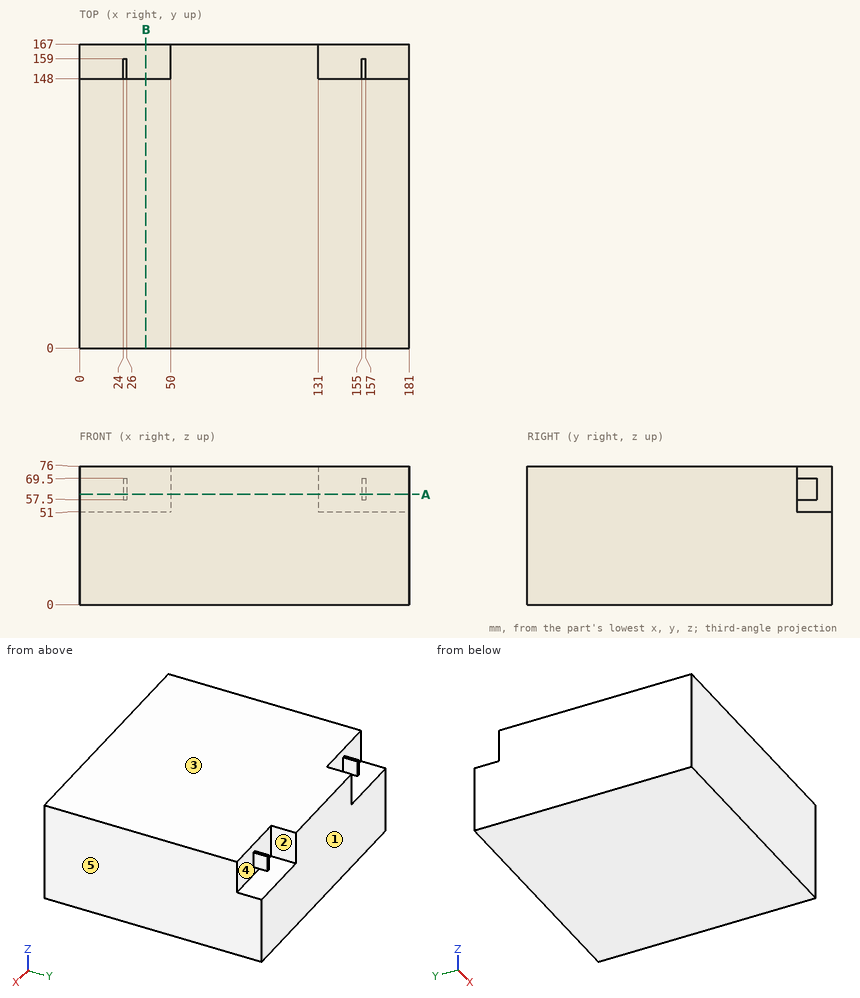
Geometry: see drawing. Coordinates: mm, zero at the bounding-box minimum. A direction names the side the tool comes from. Give positions to 0.01 mm unless a question says otherwise; leave off trailing zeros. Write each loop counter-clockwise with the first axis right and the second up, starting at its lowest first coordinate (ties: lowest second). Pieces come first, ordered by that corner, then holes. Notation, with made-up numbers: M 76,-8 L 117,-8 A17 ccw 117,-3 Z; hole C -32,-15.75 d2. An arc over 180 degrees is marked long. Return JSON: item names as keys, results as strings. Group by question number.
1) Set-up query: the marked faces 1 and 2. Return all of +Z, -Z, +X, -X, +Y, -Y with unobstructed straight access to the full face (end or side cutting, diameter ignored); none if empty.
2) Cut plane B-B, the plane x = 36.5. Output: boundary loops of the cut face in (y, z), then the cut area to 3 significant figures.
3) Ray query, L1, parallel to X at y = 156, z = 58; L2, parallel to Y at x = 21, z = 62.5. Return the intervals inside material, ascending.
4) Draft query along X for the marked faces 3, 4 and 5. Return one class per face: released by +X, released by -X, zero draft, split by the parting line, or undercut.
5) Cut plane A-A, the plane z = 60.5. Output: boundary loops of the cut face in (x, y), then the cut area to 3 significant figures.
6) First-contact query: pin 1 Ø9.5 at (x, y) = (158.5, 160) entering from +Z; pin 2 Ø5.5 at (y, z) = (152.5, 61.5) entering from +X; pin 3 Ø2 at (x, z) = (156, 61) entering from +Y. Flat tips, straight axial feed; report the tip coordinate or a pass-through.
Data:
{
 "1": {"face 1": "+Z, -Z, +X, -X, +Y", "face 2": "+Z, +Y"},
 "2": {"outline": "M 0,0 L 167,0 L 167,51 L 148,51 L 148,76 L 0,76 Z", "area": "12,200 mm²"},
 "3": {"L1": "x = 24 to 26, 50 to 131, 155 to 157", "L2": "y = 0 to 148"},
 "4": {"face 3": "zero draft", "face 4": "undercut", "face 5": "released by +X"},
 "5": {"outline": "M 0,0 L 181,0 L 181,148 L 157,148 L 157,159 L 155,159 L 155,148 L 131,148 L 131,167 L 50,167 L 50,148 L 26,148 L 26,159 L 24,159 L 24,148 L 0,148 Z", "area": "28,400 mm²"},
 "6": {"pin 1": "stops at z = 69.5", "pin 2": "stops at x = 157", "pin 3": "stops at y = 159"}
}
